```python
from build123d import *

# Parameters (mm, degrees)
F0_W     = 50.8
F0_H     = 24.7
F1_DEPTH = 0.5
F2_R     = 1.5
F3_DEPTH = 25
F5_DEPTH = 25
F6_DEPTH = 25
F7_DEPTH = 25
F9_DEPTH = 25


with BuildPart() as f1:
    # F0 (on Top) → F1 (new body, symmetric)
    with BuildSketch(Plane.XY):
        Rectangle(F0_W, F0_H)
    extrude(amount=F1_DEPTH, both=True)

    # F2 (on face) → F3 (cut)
    with BuildSketch(Plane.XY.offset(0.5)):
        with Locations((12.5349592417, -4.9380455166)):
            Circle(F2_R)
    extrude(amount=-F3_DEPTH, mode=Mode.SUBTRACT)

    # F4 (on face) → F5 (cut)
    with BuildSketch(Plane(origin=(0, 0, -0.5), x_dir=(1, 0, 0), z_dir=(0, 0, -1))):
        with BuildLine():
            ThreePointArc((-13.2667996844, 3.8108435868), (-12.1922088341, 4.2424211974), (-11.7452072576, 5.3106881678))
            ThreePointArc((-11.7452072576, 5.3106881678), (-12.1505501018, 6.3362249596), (-13.147508206, 6.8075030847))
            Line((-13.147508206, 6.8075030847), (-13.2993535533, 6.8097105755))
            Line((-13.2993535533, 6.8097105755), (-13.2452072576, 5.3106881678))
            Line((-13.2452072576, 5.3106881678), (-13.3017715787, 3.8117550547))
            ThreePointArc((-13.3017715787, 3.8117550547), (-13.2842882888, 3.8111973632), (-13.2667996844, 3.8108435868))
        make_face()
        with BuildLine():
            Line((-13.2452072576, 5.3106881678), (-13.2993535533, 6.8097105755))
            ThreePointArc((-13.2993535533, 6.8097105755), (-14.7452067697, 5.3118980046), (-13.3017715787, 3.8117550547))
            Line((-13.3017715787, 3.8117550547), (-13.2452072576, 5.3106881678))
        make_face()
    extrude(amount=-F5_DEPTH, mode=Mode.SUBTRACT)

    # F4 (on face) → F6 (cut)
    with BuildSketch(Plane(origin=(0, 0, -0.5), x_dir=(1, 0, 0), z_dir=(0, 0, -1))):
        with BuildLine():
            ThreePointArc((-13.147508206, 6.8075030847), (-12.1505501018, 6.3362249596), (-11.7452072576, 5.3106881678))
            ThreePointArc((-11.7452072576, 5.3106881678), (-12.1922088341, 4.2424211974), (-13.2667996844, 3.8108435868))
            Line((-13.2667996844, 3.8108435868), (12.4463466927, 3.4406651988))
            ThreePointArc((12.4463466927, 3.4406651988), (11.0349592417, 4.9380455166), (12.4463466927, 6.4354258344))
            Line((12.4463466927, 6.4354258344), (-13.147508206, 6.8075030847))
        make_face()
    extrude(amount=-F6_DEPTH, mode=Mode.SUBTRACT)

    # F4 (on face) → F7 (cut)
    with BuildSketch(Plane(origin=(0, 0, -0.5), x_dir=(1, 0, 0), z_dir=(0, 0, -1))):
        with BuildLine():
            ThreePointArc((12.4463466927, -1.5), (13.5070068645, -1.0606601718), (13.9463466927, 0))
            ThreePointArc((13.9463466927, 0), (13.5070068645, 1.0606601718), (12.4463466927, 1.5))
            Line((12.4463466927, 1.5), (12.4463466927, -1.5))
        make_face()
        with BuildLine():
            Line((12.4463466927, -1.5), (12.4463466927, 1.5))
            ThreePointArc((12.4463466927, 1.5), (10.9463466927, 0), (12.4463466927, -1.5))
        make_face()
        with BuildLine():
            ThreePointArc((12.4463466927, -1.5), (10.9463466927, 0), (12.4463466927, 1.5))
            Line((12.4463466927, 1.5), (-13.3017869666, 1.5))
            ThreePointArc((-13.3017869666, 1.5), (-12.2411267948, 1.0606601718), (-11.8017869666, 0))
            ThreePointArc((-11.8017869666, 0), (-12.2411267948, -1.0606601718), (-13.3017869666, -1.5))
            Line((-13.3017869666, -1.5), (12.4463466927, -1.5))
        make_face()
        with BuildLine():
            ThreePointArc((-11.8017869666, 0), (-12.2411267948, 1.0606601718), (-13.3017869666, 1.5))
            Line((-13.3017869666, 1.5), (-13.3017869666, -1.5))
            ThreePointArc((-13.3017869666, -1.5), (-12.2411267948, -1.0606601718), (-11.8017869666, 0))
        make_face()
        with BuildLine():
            Line((-13.3017869666, -1.5), (-13.3017869666, 1.5))
            ThreePointArc((-13.3017869666, 1.5), (-14.8017869666, 0), (-13.3017869666, -1.5))
        make_face()
        with BuildLine():
            ThreePointArc((12.1577924413, -7.1743104644), (13.3265385473, -6.8031241581), (13.8277874587, -5.6839743633))
            ThreePointArc((13.8277874587, -5.6839743633), (13.4095745674, -4.6448705901), (12.3881385899, -4.1851889414))
            Line((12.3881385899, -4.1851889414), (12.1577924413, -7.1743104644))
        make_face()
        with BuildLine():
            Line((12.1577924413, -7.1743104644), (12.3881385899, -4.1851889414))
            ThreePointArc((12.3881385899, -4.1851889414), (10.8322215741, -5.5687238327), (12.1577924413, -7.1743104644))
        make_face()
        with BuildLine():
            ThreePointArc((12.1577924413, -7.1743104644), (10.8322215741, -5.5687238327), (12.3881385899, -4.1851889414))
            Line((12.3881385899, -4.1851889414), (-13.0010832561, -3.162848961))
            ThreePointArc((-13.0010832561, -3.162848961), (-12.0590596608, -3.6572043001), (-11.6817944423, -4.6519236627))
            ThreePointArc((-11.6817944423, -4.6519236627), (-12.1427083133, -5.733727719), (-13.2421944641, -6.1507071151))
            Line((-13.2421944641, -6.1507071151), (12.1577924413, -7.1743104644))
        make_face()
        with BuildLine():
            ThreePointArc((-11.6817944423, -4.6519236627), (-12.0590596608, -3.6572043001), (-13.0010832561, -3.162848961))
            Line((-13.0010832561, -3.162848961), (-13.2421944641, -3.1531402102))
            Line((-13.2421944641, -3.1531402102), (-13.2421944641, -6.1507071151))
            ThreePointArc((-13.2421944641, -6.1507071151), (-12.1427083133, -5.733727719), (-11.6817944423, -4.6519236627))
        make_face()
        with BuildLine():
            ThreePointArc((-13.2421944641, -3.1531402102), (-14.6817944423, -4.6519236627), (-13.2421944641, -6.1507071151))
            Line((-13.2421944641, -6.1507071151), (-13.2421944641, -3.1531402102))
        make_face()
    extrude(amount=-F7_DEPTH, mode=Mode.SUBTRACT)

    # F8 (on face) → F9 (cut)
    with BuildSketch(Plane(origin=(0, 0, -0.5), x_dir=(1, 0, 0), z_dir=(0, 0, -1))):
        Polygon((8.5604507476, 10.399765335), (9.3251494691, 12.3484628275), (9.31405598, 12.35), (7.7857054425, 12.35), align=None)
        Polygon((6.7462604493, 10.399765335), (7.2912084784, 12.35), (6.2853197637, 12.35), align=None)
        Polygon((5.3150104359, 10.4954689741), (5.8871536403, 12.35), (4.7833247403, 12.35), align=None)
        Polygon((4.5080462822, 12.35), (3.6044052231, 12.35), (4.3411315419, 10.4954689741), align=None)
    extrude(amount=-F9_DEPTH, mode=Mode.SUBTRACT)


solid = f1.part
```
For this review, take the finished solid that the model builds, in its own axes (mm). A direction names the side the tool comes from. Give positions to 0.01 mm unless a question says otherwise; leave off trailing zeros. Write each loop counter-clockwise with the first axis right and the second up, starting at its lowest first coordinate (ties: lowest second). Pieces come first, ordered by that corner, then holes.
Item 1: Take a section at B-B (x = -9). Give the boundary of the cut face in (y, z).
Item 2: Wall thickness on probe 1 along Y at (x, z) = (12.5, 0.05); probe 2 along Y at (x, z) = (-14.5, 0.4); probe 3 along X at (y, z) = (-11, -0.1): over which ranges is each line inside the solid? List them lowest first.
Item 3: Machinability: for faces 1 (the face through (0, -1.5, 0)), 2 (the face through (0, 3, 0.5)), which of the approach directions +Z, -Z, +X, -X, +Y, -Y give a long, thin tool a straight path to every point of the face, cutting with its end or side? Answer none if there is none.
Item 4: The part is to be moulded in two halves that separate along X. For faces 3 (the face through (17, -12.35, 0)), 4 (the face through (25.4, 0, 0)), 5 (the face through (4.423, -11.41, -0.007)), 6 (the face through (3.968, -11.436, -0.007)), say which applies: +X half, -X half, draft (parallel to the pull), parting line (faces both ways), or undercut.
Item 5: Take a section at A-A (z = 0.1). Give the number of separate pieces and of enclosed holes in the cut face, and give its area (3 significant figures).
Item 6: Take a section at C-C (y = 1). Give the boundary of the cut face in (x, z).
Established:
1. outline: (-12.35, -0.5) - (-6.75, -0.5) - (-6.75, 0.5) - (-12.35, 0.5) - close; (-3.75, -0.5) - (-1.5, -0.5) - (-1.5, 0.5) - (-3.75, 0.5) - close; (1.5, -0.5) - (3.32, -0.5) - (3.32, 0.5) - (1.5, 0.5) - close; (6.32, -0.5) - (12.35, -0.5) - (12.35, 0.5) - (6.32, 0.5) - close
2. probe 1: y = -12.35 to -6.44, -3.44 to -1.5, 1.5 to 4.19, 7.17 to 12.35
2. probe 2: y = -12.35 to -6.13, -4.49 to -0.9, 0.9 to 3.94, 5.37 to 12.35
2. probe 3: x = -25.4 to 4.14, 4.39 to 5.17, 5.47 to 6.6, 6.91 to 8.32, 8.8 to 25.4
3. face 1: +Z, -Z
3. face 2: +Z, +X, -X, +Y, -Y
4. face 3: draft
4. face 4: +X half
4. face 5: undercut
4. face 6: undercut
5. separate pieces: 1
5. enclosed holes: 3
5. area: 998 mm2
6. outline: (-25.4, -0.5) - (-14.42, -0.5) - (-14.42, 0.5) - (-25.4, 0.5) - close; (13.56, -0.5) - (25.4, -0.5) - (25.4, 0.5) - (13.56, 0.5) - close
